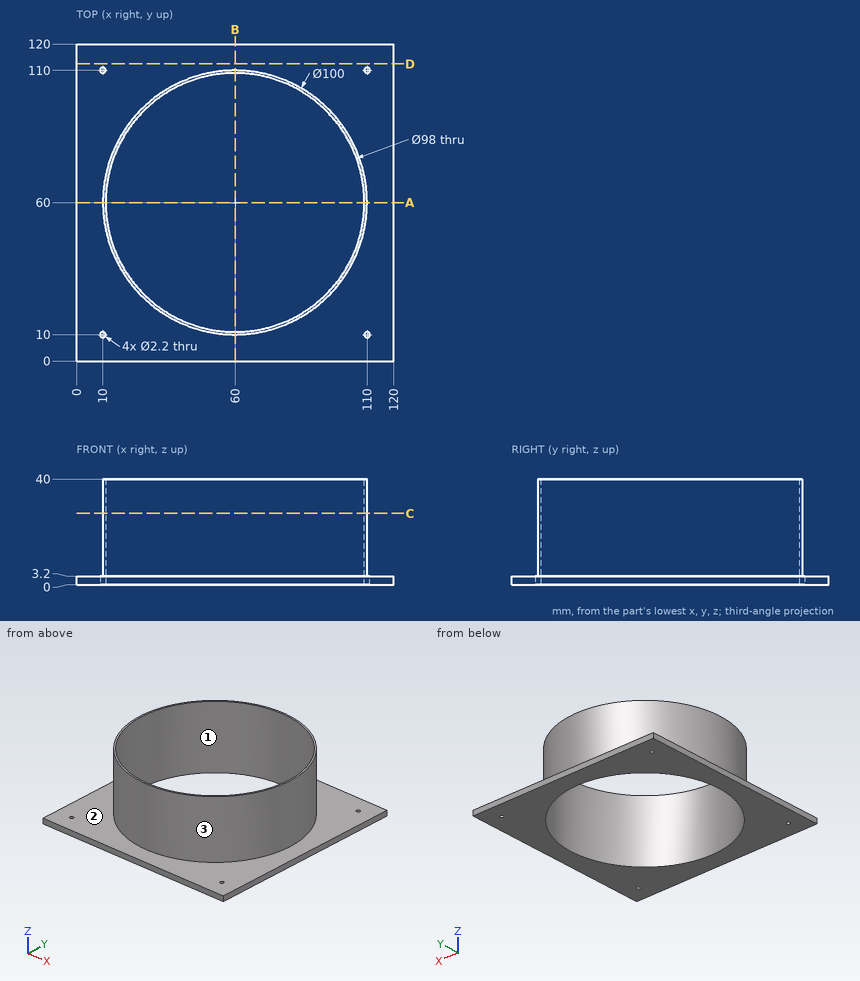
Check sheet for the drawn part. Datum: minimum x, y, z corner. Units: mm. Round coordinates to 2 decimals unless told otherwise and drop trailing zeros. Write each loop counter-clockwise with the first axis right and the second up, starting at its lowest first coordinate (ties: lowest second). Pieces come first, ordered by that corner, then holes. Notation, with made-up numbers: (70, -23) -> (128, -23) arc R29 ccw to (128, 14) -> close; hole circle Ø10 at (28.5, -29.75). An arc over 180 degrees is marked (long way). Write each question's results on one line, items separated by ' | '. Start each with the question number.
1. Depth check by flat-ended pin: P1, Ø1.5, axis at x = 75, z = 33.5, coming from the +Y side; P2, Ø3.5, axis at x = 10, y = 110, coming from the +Z side; P3, Ø2, axis at x = 29, z = 26.5, coming from the +Y side. Enter the tip coordinate at first touch or a pass-through.
2. Cross-section at A-A (y = 60). Enter the section's corners in (x, z).
3. Cross-section at C-C (z = 27). Enter the section's corners in (x, y), then the cut area to 3 significant figures.
4. Draft check along Y on the marked faces 1, 2 and 3. Enter one of: +Y half, -Y half, draft (parallel to the pull), parting line (faces both ways), or undercut.
5. Cross-section at D-D (y = 112.5). Enter the section's corners in (x, z), then the cut area to 3 significant figures.
6. Material ranges on probe 1 along X at (y, z) = (110, 2); probe 2 along Y at (x, z) = (60, 15), recorded low to high. Write a range as from..to.
Solutions:
1) P1: stops at y = 107.93 | P2: stops at z = 3.2 | P3: stops at y = 100
2) outline: (0, 0) -> (11, 0) -> (11, 40) -> (10, 40) -> (10, 3.2) -> (0, 3.2) -> close; (109, 0) -> (120, 0) -> (120, 3.2) -> (110, 3.2) -> (110, 40) -> (109, 40) -> close
3) outline: circle Ø100 at (60, 60); hole circle Ø98 at (60, 60) | area: 311 mm2
4) face 1: undercut | face 2: draft | face 3: parting line
5) outline: (0, 0) -> (120, 0) -> (120, 3.2) -> (0, 3.2) -> close | area: 384 mm2
6) probe 1: x = 0..8.9, 11.1..108.9, 111.1..120 | probe 2: y = 10..11, 109..110
